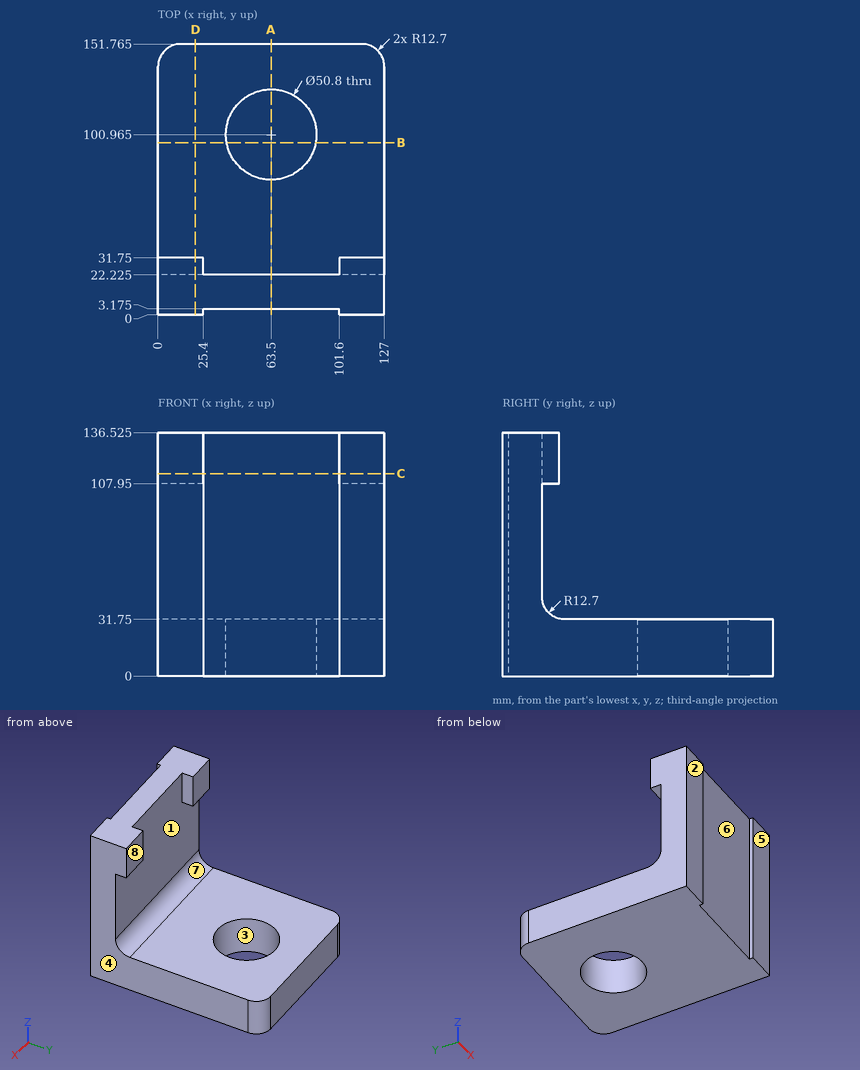
Design review of the part shown in the three views and the two pictorial views. Dimensions are in mm from the part's minimum x, y and z. A direction names the side the tool comes from. Round coordinates to 2 decimals unless told otherwise and drop trailing zeros. Order: outer loops, then holes, each group sorted by start corner. A loop starts at its lowest first (then second) coordinate and runs counter-clockwise, first axis right, second up. Notation, with made-up numbers: (-40, 40) - (-3, 40) arc R5 ccw to (-3, 49) - close; hole circle Ø4 at (-11, -30). An arc over 180 degrees is marked (long way). One line per question, with ' | ' between items.
Item 1: Take a section at A-A, the plane x = 63.5. Write out the cut boundary in (y, z) (3 decimals).
Checks:
outline: (3.175, 0) - (75.565, 0) - (75.565, 31.75) - (34.925, 31.75) arc R12.7 cw to (22.225, 44.45) - (22.225, 136.525) - (3.175, 136.525) - close; (126.365, 0) - (151.765, 0) - (151.765, 31.75) - (126.365, 31.75) - close
Item 2: Take a section at B-B, the plane y = 96.5. Write out the cut boundary in (x, z).
Checks:
outline: (0, 0) - (38.5, 0) - (38.5, 31.75) - (0, 31.75) - close; (88.5, 0) - (127, 0) - (127, 31.75) - (88.5, 31.75) - close
Item 3: Wall thickness on line 1 (Y direction, x = 63.5, z = 18.5) (3 decimals); line 2 (Z direction, x = 42, y = 115); line 3 (Y direction, x = 56.5, z = 25.5) (3 decimals): over which ranges is each line inside the solid? List them lowest first. Write a range as [from, to].
Checks:
line 1: [3.175, 75.565], [126.365, 151.765] | line 2: [0, 31.75] | line 3: [3.175, 76.549], [125.381, 151.765]
Item 4: For P1, Ø1, axis at x = 37.5, z = 42, coming from the -Y side (3 decimals); P2, Ø5, axis at x = 10.5, y = 28.5, coming from the -Z side; P3, Ø1.5, axis at x = 78.5, z = 36.5, coming from the +Y side; P4, Ø7.5, axis at x = 12, z = 123, coming from the +Y side, all flat-tipped, find the tip position at first contact; note any pin that passes through.
Checks:
P1: y = 3.175 | P2: z = 0 | P3: y = 25.67 | P4: y = 31.75
Item 5: Take a section at D-D, the plane x = 21. Write out the cut boundary in (y, z) (3 decimals), then the cut area to 3 significant figures.
Checks:
outline: (0, 0) - (151.765, 0) - (151.765, 31.75) - (34.925, 31.75) arc R12.7 cw to (22.225, 44.45) - (22.225, 107.95) - (31.75, 107.95) - (31.75, 136.525) - (0, 136.525) - close | area: 7,450 mm²
Item 6: Machinability: for the marked faces 5, 6, 7 and 8, which of the approach directions +Z, -Z, +X, -X, +Y, -Y give a long, thin tool a straight path to every point of the face, cutting with its end or side? Answer none if there is none.
Checks:
face 5: +Z, -Z, +X, -X, -Y | face 6: +Z, -Z, -Y | face 7: +X, -X, +Y | face 8: +Z, +X, -X, +Y
Item 7: Take a section at C-C, the plane z = 113.5. Write out the cut boundary in (x, y) (3 decimals), then the cut area to 3 significant figures.
Checks:
outline: (0, 0) - (25.4, 0) - (25.4, 3.175) - (101.6, 3.175) - (101.6, 0) - (127, 0) - (127, 31.75) - (101.6, 31.75) - (101.6, 22.225) - (25.4, 22.225) - (25.4, 31.75) - (0, 31.75) - close | area: 3,060 mm²
Item 8: Draft analysis for pull direction X (two halves, no side actions). For the marked faces 1, 2, 3 and 4, state which applies: +X half, -X half, draft (parallel to the pull), parting line (faces both ways), or undercut.
Checks:
face 1: undercut | face 2: draft | face 3: undercut | face 4: +X half
